Could you check a few things on this model? Use its own coordinates, in mm. A direction names the side the tool comes from. Give positions to 0.01 mm unless a question says otherwise; leave off trailing zeros. Order: outer loops, then holes, each group sorted by start corner. A loop starts at its lowest first (then second) coordinate and runs counter-clockwise, first axis right, second up.
(1) If we mould it in two halves opening along Y, with no side actions, what happens to faces 1 (the flat face through (0, 14, -17.15)), 2 (the cylindrical face through (-1.107, 18.328, -13.571)), 3 (the flat face through (0, 28, 0)), 4 (the flat face through (5, 17, -15.05))? For each: released by +Y, released by -Y, zero draft, split by the parting line, or undercut.
(2) Imagine slicing it at C-C, the plane z = 0. Write out the boundary of the cut face in (x, y), then the cut area to 3 significant figures.
(3) Imagine slicing it at B-B, the plane z = 6. Write out the boundary of the cut face in (x, y), then the cut area to 3 significant figures.
(4) Will these pins go through, and if not, where does the flat tip stop? pin 1 (6.5 mm diameter, centred on x = -6, z = 0, fed in from -Y); pin 2 (8 mm diameter, centred on x = 0, z = -13.5, fed in from -Y); pin 3 (3.5 mm diameter, centred on x = 6, y = 9.9, fed in from +Z).
(5) Imagine slicing it at A-A, the plane y = 22. Write out the boundary of the cut face in (x, z).
(6) Imagine slicing it at D-D, the plane x = 6. Write out the boundary of the cut face in (y, z).
(7) On a 3-axis mill with a long thin cutter (end or side, diameter ignored), from which of +Z, -Z, +X, -X, +Y, -Y can I reach the whole of each face in a straight line? I mean faces 5 (the flat face through (2, 8, -12.05)), 6 (the cylindrical face through (-0.26, 5.883, 16.115)), 7 (the cylindrical face through (-7.6, 26, -1.2)). Say none if no direction works.
(8) If I drill on probe 1 along Y at (x, z) = (0, 15.6); probe 2 along Z at (x, y) = (6, 25.5); probe 3 along Z at (x, y) = (8.25, 6), over which ranges is the centre line in solid material (lowest first)?
from build123d import *

# Parameters (mm, degrees)
F0_W     = 4
F0_H     = 30.1
F0_H_2   = 2.1
F0_W_2   = 24
F1_DEPTH = 9.9
F3_DEPTH = 34.301
F2_R     = 2
F4_DEPTH = 2.1
F5_R     = 8.5
F5_R_2   = 2
F6_DEPTH = 3
F7_DEPTH = 2.101
F8_R     = 2
F9_DEPTH = 4.001


with BuildPart() as f1:
    # F0 (on Right) → F1 (new body, symmetric)
    with BuildSketch(Plane.YZ):
        Polygon((28, 17.15), (0, 17.15), (0, 15.05), (24, 15.05), (28, 15.05), align=None)
        with Locations((26, 0)):
            Rectangle(F0_W, F0_H)
        with Locations((26, -16.1)):
            Rectangle(F0_W, F0_H_2)
        with Locations((12, -16.1)):
            Rectangle(F0_W_2, F0_H_2)
    extrude(amount=F1_DEPTH, both=True)

    # F2 (on face) → F3 (cut, through all)
    with BuildSketch(Plane.XY.offset(17.15)):
        Polygon((-9.9, 0), (-9.9, 9.9), (-14.9, 9.9), (-14.9, -5), (14.9, -5), (14.9, 9.9), (9.9, 9.9), (9.9, 0), (0, 0), align=None)
        with BuildLine():
            ThreePointArc((0, 0), (-7.000357, 2.899643), (-9.9, 9.9))
            Line((-9.9, 9.9), (-9.9, 0))
            Line((-9.9, 0), (0, 0))
        make_face()
        with BuildLine():
            ThreePointArc((9.9, 9.9), (7.000357, 2.899643), (0, 0))
            Line((0, 0), (9.9, 0))
            Line((9.9, 0), (9.9, 9.9))
        make_face()
    extrude(amount=-F3_DEPTH, mode=Mode.SUBTRACT)

    # F2 (on face) → F4 (cut, through all)
    with BuildSketch(Plane.XY.offset(17.15)):
        with Locations((-6, 9.9)):
            Circle(F2_R)
        with Locations((0, 15.9)):
            Circle(F2_R)
        with Locations((6, 9.9)):
            Circle(F2_R)
        with Locations((0, 3.9)):
            Circle(F2_R)
    extrude(amount=-F4_DEPTH, mode=Mode.SUBTRACT)

    # F5 (on face) → F6 (join)
    with BuildSketch(Plane.XY.offset(-15.05)):
        with Locations((0, 9.9)):
            Circle(F5_R)
        with Locations((0, 9.9)):
            Circle(F5_R_2, mode=Mode.SUBTRACT)
    extrude(amount=F6_DEPTH)

    # F5 (on face) → F7 (cut, through all)
    with BuildSketch(Plane.XY.offset(-15.05)):
        with Locations((0, 9.9)):
            Circle(F5_R_2)
    extrude(amount=-F7_DEPTH, mode=Mode.SUBTRACT)

    # F8 (on face) → F9 (cut, through all)
    with BuildSketch(Plane.XZ.offset(-24)):
        with Locations((0, 6)):
            Circle(F8_R)
        with Locations((6, 0)):
            Circle(F8_R)
        with Locations((0, -6)):
            Circle(F8_R)
        with Locations((-6, 0)):
            Circle(F8_R)
    extrude(amount=-F9_DEPTH, mode=Mode.SUBTRACT)


solid = f1.part
Answer block:
1. face 1: zero draft
1. face 2: undercut
1. face 3: released by +Y
1. face 4: undercut
2. outline: (-9.9, 24) - (-8, 24) - (-8, 28) - (-9.9, 28) - close; (-4, 24) - (4, 24) - (4, 28) - (-4, 28) - close; (8, 24) - (9.9, 24) - (9.9, 28) - (8, 28) - close
2. area: 47.2 mm2
3. outline: (-9.9, 24) - (-2, 24) - (-2, 28) - (-9.9, 28) - close; (2, 24) - (9.9, 24) - (9.9, 28) - (2, 28) - close
3. area: 63.2 mm2
4. pin 1: stops at y = 24
4. pin 2: stops at y = 0
4. pin 3: stops at z = -12.05
5. outline: (-9.9, -17.15) - (9.9, -17.15) - (9.9, -15.05) - (-9.9, -15.05) - close; (-9.9, 15.05) - (9.9, 15.05) - (9.9, 17.15) - (-9.9, 17.15) - close
6. outline: (2.03, -17.15) - (28, -17.15) - (28, -2) - (24, -2) - (24, -15.05) - (15.92, -15.05) - (15.92, -12.05) - (3.88, -12.05) - (3.88, -15.05) - (2.03, -15.05) - close; (2.03, 15.05) - (7.9, 15.05) - (7.9, 17.15) - (2.03, 17.15) - close; (11.9, 15.05) - (24, 15.05) - (24, 2) - (28, 2) - (28, 17.15) - (11.9, 17.15) - close
7. face 5: +X, -X, -Y
7. face 6: +Z
7. face 7: +Y, -Y
8. probe 1: y = 0 to 1.9, 5.9 to 13.9, 17.9 to 28
8. probe 2: z = -17.15 to -2, 2 to 17.15
8. probe 3: z = -17.15 to -15.05, 15.05 to 17.15
